Check sheet for the modelled part. Datum: model origin and axes. Units: mm. A direction names the side the tool comes from. Round coordinates to 2 decimals unless told otherwise and drop trailing zeros. Write each loop counter-clockwise with the first axis right and the second up, starting at its lowest first coordinate (ties: lowest second). Pieces come first, ordered by that corner, then holes. Notation, with made-up numbers: (-11, 12) -> (10, 12) arc R13 ccw to (10, 22) -> close; hole circle Ø1 at (32, 88). An arc over 180 degrees is marked (long way). One line per item, written item: value.
Autodesk Inventor part; units mm, degrees
ref_plane "Work Plane1" through (0, 25, 0) normal (0, 1, 0) x (-1, 0, 0)
ref_plane "YZ Plane" through (0, 0, 0) normal (1, 0, 0) x (0, 1, 0)
ref_plane "XY Plane" through (0, 0, 0) normal (0, 0, 1) x (1, 0, 0)
sketch "Sketch1" plane through (0, 0, 0) normal (0, 0, 1) x (1, 0, 0)
  circle A0 centre (0, 0) radius 25
  circle A1 centre (0, -13) radius 1.65
  circle A2 centre (-9, 10) radius 1.65
  circle A3 centre (9, 10) radius 1.65
  circle A4 centre (-9, 10) radius 3
  circle A5 centre (9, 10) radius 3
  circle A6 centre (0, -13) radius 3
  dimension "d0" = 50
  dimension "d1" = 13
  dimension "d2" = 10
  dimension "d3" = 9
  dimension "d4" = 9
  dimension "d5" = 3.3
  dimension "d6" = 6
extrude "Extrusion1" add sketch "Sketch1" along normal blind 5 contours A0
extrude "Extrusion2" add sketch "Sketch1" along normal blind 10 contours A4 | A5 | A6
sketch "Sketch2" plane through (0, 0, 0) normal (0, 0, -1) x (-1, 0, 0)
  circle A0 centre (0, -13) radius 1.65
  circle A1 centre (-9, 10) radius 1.65
  circle A2 centre (9, 10) radius 1.65
  circle A3 centre (0, 0) radius 25
  circle A4 centre (-9, 10) radius 3.5
  circle A5 centre (9, 10) radius 3.5
  circle A6 centre (0, -13) radius 3.5
  dimension "d11" = 7
extrude "Extrusion3" cut sketch "Sketch2" against normal blind 3 contours A4 | A5 | A6
chamfer "Chamfer1" distance 1.8199 angle 70 3 edges at (-3, -13, 5) (-12, 10, 5) (6, 10, 5) measured on face at (12.0972, -3.5223, 5)
chamfer "Chamfer2" distance 2 angle 45 1 edges at (-25, 0, 5)
sketch "Sketch3" plane through (0, 0, 0) normal (1, 0, 0) x (0, 1, 0)
  line L0 (14.8199, 5) -> (5.1801, 5)
  line L1 (-8.1801, 5) -> (-17.8199, 5)
  line L2 (14.8199, 5) -> (5.1801, 5)
  line L3 (-23, 5) -> (23, 5)
  line L4 (25, 0) -> (25, 3)
  line L5 (25, 3) -> (-25, 3)
  line L6 (-23, 5) -> (23, 5)
  line L7 (25, 3) -> (23, 5)
  arc A0 (18.1033, 14) -> (23, 5) centre (28.8225, 14) ccw
  line L8 (18.1033, 14) -> (17.1033, 14)
  line L9 (17.1033, 14) -> (17.1033, 5)
  line L10 (0, -3.8) -> (0, 22.8)
  point P0 (0, 0)
  dimension "d20" = 9
  dimension "d21" = 18.1033
  dimension "d22" = 1
revolve "Revolution1" add sketch "Sketch3" angle 360 about axis through (0, 0, -10) along (0, 0, 1) contours L9 L8 A0 L3
sketch "Sketch5" plane through (0, 0, 14) normal (0, 0, 1) x (1, 0, 0)
  line L0 (4, 17.5) -> (-4, 17.5)
  line L1 (-4, 17.5) -> (-7, 16)
  line L2 (-7, 16) -> (7, 16)
  line L3 (7, 16) -> (4, 17.5)
  point P0 (0, 0)
  point P1 (0, 16)
  point P2 (0, 17.5)
  dimension "d37" = 16
  dimension "d39" = 14
  dimension "d42" = 8
  dimension "d43" = 1.5
extrude "Extrusion6" add sketch "Sketch5" against normal up to surface (9 mm away)
ref_plane "Work Plane1" through (0, 25, 0) normal (0, 1, 0) x (-1, 0, 0)
sketch "Sketch4" plane through (0, 25, 0) normal (0, 1, 0) x (-1, 0, 0)
  line L0 (-8.5709, 5) -> (-6.0434, 5)
  line L1 (13.8192, 5) -> (8.5709, 5)
  line L2 (13.8192, 5) -> (2.8899, 5)
  line L3 (-2.8899, 5) -> (2.8899, 5)
  line L4 (-2.8899, 5) -> (-13.8192, 5)
  line L5 (-8.5709, 5) -> (-13.8192, 5)
  line L6 (-2.5, 8.5) -> (2.5, 8.5) construction
  line L7 (3.5, 3) -> (-3.5, 3)
  line L8 (-2.5, 5.25) -> (2.5, 5.25)
  line L9 (2.5, 11.75) -> (-2.5, 11.75)
  arc A0 (-2.5, 11.75) -> (-2.5, 5.25) centre (-2.5, 8.5) ccw
  arc A1 (2.5, 5.25) -> (2.5, 11.75) centre (2.5, 8.5) ccw
  line L10 (-3, 8.5) -> (3, 8.5) construction
  line L11 (-3, 7) -> (3, 7)
  line L12 (3, 10) -> (-3, 10)
  arc A2 (-3, 10) -> (-3, 7) centre (-3, 8.5) ccw
  arc A3 (3, 7) -> (3, 10) centre (3, 8.5) ccw
  line L13 (-6.0434, 5) -> (6.0434, 5)
  line L14 (6.0434, 5) -> (8.5709, 5)
  point P0 (0, 0)
  point P1 (0, 5)
  point P2 (0, 8.5)
  point P3 (0, 5)
  point P4 (0, 8.5)
  dimension "d30" = 6.5
  dimension "d31" = 11.5
  dimension "d32" = 3.5
  dimension "d33" = 3
  dimension "d34" = 9
extrude "Extrusion4" cut sketch "Sketch4" against normal blind 10 contours A2 L12 A3 L11
extrude "Extrusion5" cut sketch "Sketch4" against normal blind 8
sketch "Sketch7" plane through (0, 0, 5) normal (0, 0, 1) x (1, 0, 0)
  line L0 (-15, 5) -> (15, 5)
  line L1 (15, 5) -> (15, -5)
  line L2 (15, -5) -> (-15, -5)
  line L3 (-15, -5) -> (-15, 5)
  point P0 (0, 0)
  point P1 (0, 5)
  point P2 (-15, 0)
  dimension "d50" = 30
  dimension "d51" = 10
extrude "Extrusion8" cut sketch "Sketch7" against normal through all
sketch "Sketch8" plane through (0, 0, 0) normal (0, 0, -1) x (-1, 0, 0)
  line L0 (27, 6.75) -> (15, 6.75)
  line L1 (15, 6.75) -> (15, -6.75)
  line L2 (15, -6.75) -> (27, -6.75)
  line L3 (27, -6.75) -> (27, 6.75)
  point P0 (0, 0)
  point P1 (15, 5)
  point P2 (15, 0)
  dimension "d54" = 13.5
  dimension "d55" = 12
extrude "Extrusion9" cut sketch "Sketch8" against normal blind 2.7
chamfer "Chamfer3" distance 1.75 angle 45 2 edges at (-15, 5, 1.35) (-15, -5, 1.35)
properties part number "Baseplate"
Item 1: Sectioned sample at C-C on z = 6. Enter the section's corners in (x, y), and give its area (3 significant figures).
Answer:
outline: (-4.58, 17) -> (-4.58, 21.2) arc R21.69 ccw (long way) to (4.58, 21.2) -> (4.58, 17) -> close; hole (-13.41, 10.61) arc R17.1 ccw to (-1.99, -16.99) arc R4.46 cw (long way) to (1.99, -16.99) arc R17.1 ccw to (13.41, 10.61) arc R4.46 cw (long way) to (9.14, 14.45) arc R17.1 ccw to (6.04, 16) -> (-6.04, 16) arc R17.1 ccw to (-9.14, 14.45) arc R4.46 cw (long way) to start; hole circle Ø3.3 at (-9, 10); hole circle Ø3.3 at (0, -13); hole circle Ø3.3 at (9, 10)
area: 680 mm^2
Item 2: Sectioned sample at B-B on y = 0. Enter the section's corners in (x, z).
Answer:
outline: (-25, 2.7) -> (-15, 2.7) -> (-15, 5) -> (-17.1, 5) -> (-17.1, 14) -> (-18.1, 14) arc R10.72 cw to (-23, 5) -> (-25, 3) -> close; (15, 0) -> (25, 0) -> (25, 3) -> (23, 5) arc R10.72 cw to (18.1, 14) -> (17.1, 14) -> (17.1, 5) -> (15, 5) -> close
Item 3: Sectioned sample at D-D on x = 0. Count the separate pieces of the cut face and the enclosed holes in it, and give its area (3 significant figures).
Answer:
separate pieces: 4
enclosed holes: 0
area: 222 mm^2
Item 4: Depth check by flat-ended pin: P1, Ø6.5, axis at x = 1, y = -12.5, coming from the +Z side; P2, Ø3, axis at x = -19.5, z = 2, coming from the -Y side; P3, Ø3, axis at x = 5, z = 11, coming from the +Y side; P4, Ø1.8, axis at x = -9.5, y = 9.5, coming from the +Z side. Enter the tip coordinate at first touch or a pass-through.
Answer:
P1: stops at z = 10
P2: stops at y = -17.35
P3: stops at y = 18.22
P4: passes through
Item 5: Mould release check, pull along X, two halves, no side actions. Record for faces 4 (the flat face through (-14.14, -5.89, 1.33)), 5 (the flat face through (-20, 6.75, 1)), 6 (the cylindrical face through (23.846, -7.509, 1.479)), 7 (the cylindrical face through (-4.5, 16.5, 8.5)): pulls with the +X half, pulls with the -X half, needs draft (parallel to the pull), parting line crosses it, or undercut.
Answer:
face 4: pulls with the -X half
face 5: needs draft
face 6: parting line crosses it
face 7: undercut
Item 6: Sectioned sample at A-A on z = 8.75. Enter the section's corners in (x, y), and give its area (3 significant figures).
Answer:
outline: circle Ø6.91 at (-9, 10); (-6.04, 16) -> (-4.48, 16) -> (-4.48, 17) -> (-5.74, 17) -> (-5.74, 18.61) arc R19.48 ccw (long way) to (5.74, 18.61) -> (5.74, 17) -> (4.48, 17) -> (4.48, 16) -> (6.04, 16) arc R17.1 cw (long way) to start; circle Ø6.91 at (0, -13); circle Ø6.91 at (9, 10); hole circle Ø3.3 at (-9, 10); hole circle Ø3.3 at (0, -13); hole circle Ø3.3 at (9, 10)
area: 334 mm^2
Item 7: Thickness scan on line 1 (Y direction, x = 0, z = 1.8); line 2 (Y direction, x = -6, z = 7.5); line 3 (Y direction, x = 9, z = 6.5). Record the ranges inside material, lowest first.
Answer:
line 1: y = -25 to -16.5, -9.5 to -5, 5 to 25
line 2: y = -19.39 to -16.02, 7.49 to 12.51, 16 to 19.39
line 3: y = -19.16 to -14.54, 5.73 to 8.35, 11.65 to 14.27, 14.54 to 19.16
Item 8: Tool access check on faces 1 (the flat face through (-7.7, 8.7, 10)), 2 (the flat face through (-14.14, 5.89, 1.37)), 3 (the cylindrical face through (-6.2, 7.9, 1.5)). Record the directions out of +Z, -Z, +X, -X, +Y, -Y that give a thin tool (end or side, any length) a straight path to the whole face; none if there is none.
Answer:
face 1: +Z
face 2: -Z, -X
face 3: -Z
